Could you check a few things on this model? Use its own coordinates, in mm. A direction names the side the tool comes from. Round coordinates to 2 decimals unless told otherwise and drop trailing zeros. Order: outer loops, then holes, each group sorted by start corner. A loop starts at its lowest first (then second) coordinate and runs counter-clockwise, first axis right, second up. Notation, with made-up numbers: (5.25, 81) - (17.25, 81) arc R33 cw to (17.25, 113) - close; hole circle Ø3 at (59.5, 16). An arc over 180 degrees is marked (long way). Use one line per item in the form item = value.
from build123d import *

# Parameters (mm, degrees)
F0_R      = 5
F1_DEPTH  = 60
F3_W      = 309.3655258417
F3_H      = 284.4564542174
F4_DEPTH  = 37.5
F5_SIZE   = 12
F7_DEPTH  = 75
F9_R      = 20
F11_DEPTH = 86.9450472691
F8_R      = 5
F7_FACE_R = 5
F12_DEPTH = 22.5


# Not quite as in the source:
# - a feature names something its author has since deleted; it is built from what else it names


with BuildPart() as f1:
    # F0 (on Right) → F1 (new body, symmetric)
    with BuildSketch(Plane.YZ):
        Polygon((75, 130), (-75, 130), (-90, 130), (-108.526711476, 17.9430459013), (-58.9007476441, -170), (58.9007476441, -170), (108.526711476, 17.9430459013), (90, 130), align=None)
        with Locations((0, -117.917008698)):
            Circle(F0_R, mode=Mode.SUBTRACT)
        Circle(F0_R, mode=Mode.SUBTRACT)
    extrude(amount=F1_DEPTH, both=True)

    # F3 (on face) → F4 (cut, symmetric)
    with BuildSketch(Plane.YZ):
        with Locations((9.2283859849, -86.6799689829)):
            Rectangle(F3_W, F3_H)
    extrude(amount=F4_DEPTH, both=True, mode=Mode.SUBTRACT)

    # F5
    f5_edges = [f1.edges().sort_by_distance(p)[0] for p in [
        (-60, -99.263356, 73.971523),
        (-60, 99.263356, 73.971523),
        (60, -99.263356, 73.971523),
        (60, 99.263356, 73.971523),
    ]]
    chamfer(f5_edges, length=F5_SIZE)

    # F6 (on face) → F7 (join, through all)
    with BuildSketch(Plane.YZ.offset(-37.5)):
        Polygon((92.4365120253, -42.9936263649), (-92.4365120253, -42.9936263649), (-80.5341079321, -88.0703141729), (80.5341079321, -88.0703141729), align=None)
    extrude(amount=F7_DEPTH)

    # F9
    f9_edges = [f1.edges().sort_by_distance(p)[0] for p in [
        (-37.5, 0, 55.548258),
        (37.5, 0, 55.548258),
        (-37.5, 0, -42.993626),
        (37.5, 0, -42.993626),
    ]]
    fillet(f9_edges, radius=F9_R)

    # F10 (on face) → F11 (cut, through all)
    with BuildSketch(Plane.XY.offset(130)):
        Polygon((36.0373817384, 65.5976682901), (0, 65.5976682901), (-36.0373817384, 65.5976682901), (-36.0373817384, 0), (-36.0373817384, -65.5976682901), (0, -65.5976682901), (36.0373817384, -65.5976682901), (36.0373817384, 0), align=None)
    extrude(amount=-F11_DEPTH, mode=Mode.SUBTRACT)

    # F8 (on face) + F7_face (on face) → F12 (cut, through all)
    with BuildSketch(Plane.YZ.offset(60)):
        Polygon((25.2734031528, -88.0703141729), (-80.5341079321, -88.0703141729), (-58.9007476441, -170), (25.2734031528, -170), align=None)
        with Locations((0, -117.917008698)):
            Circle(F8_R, mode=Mode.SUBTRACT)
    with BuildSketch(Plane(origin=(37.5, 0, -126.978888881), x_dir=(0, -1, 0), z_dir=(-1, 0, 0))):
        Polygon((-80.5341079321, 38.9085747081), (-58.9007476441, -43.021111119), (58.9007476441, -43.021111119), (80.5341079321, 38.9085747081), align=None)
        with Locations((0, 9.061880183)):
            Circle(F7_FACE_R, mode=Mode.SUBTRACT)
    extrude(amount=-F12_DEPTH, dir=(1, 0, 0), mode=Mode.SUBTRACT)


solid = f1.part
Item 1: Imagine slicing it at B-B on y = 0. Please give me the cut outline in (x, z), plus the area to 3 significant figures.
Found:
outline = (-60, -170) - (-37.5, -170) - (-37.5, -122.92) - (-60, -122.92) - close; (-60, -112.92) - (-37.5, -112.92) - (-37.5, -88.07) - (60, -88.07) - (60, -5) - (37.5, -5) - (37.5, -22.99) arc R20 cw to (17.5, -42.99) - (-17.5, -42.99) arc R20 cw to (-37.5, -22.99) - (-37.5, -5) - (-60, -5) - close; (-60, 5) - (-37.5, 5) - (-37.5, 35.55) arc R20 cw to (-36.04, 43.06) - (-36.04, 130) - (-60, 130) - close; (36.04, 43.06) arc R20 cw to (37.5, 35.55) - (37.5, 5) - (60, 5) - (60, 130) - (36.04, 130) - close
area = 14,800 mm2
Item 2: I need wall thicknesses on L1, parallel to Z at x = -53.75, y = 0; L2, parallel to X at y = -5.5, z = 2; L3, parallel to X at y = -33, z = 48.5. Which ranges of each line are inside material? Lowest first, please.
Found:
L1 = -170 to -122.92, -112.92 to -5, 5 to 130
L2 = -60 to -37.5, 37.5 to 60
L3 = -60 to -36.04, 36.04 to 60
Item 3: Imagine slicing it at C-C on z = 0. Please give me the cut outline in (x, y), plus the area to 3 significant figures.
Found:
outline = (-60, -99.33) - (-55.6, -103.79) - (-37.5, -103.79) - (-37.5, -5) - (-60, -5) - close; (-60, 5) - (-37.5, 5) - (-37.5, 103.79) - (-55.6, 103.79) - (-60, 99.33) - close; (37.5, -103.79) - (55.6, -103.79) - (60, -99.33) - (60, -5) - (37.5, -5) - close; (37.5, 5) - (60, 5) - (60, 99.33) - (55.6, 103.79) - (37.5, 103.79) - close
area = 8,850 mm2
Item 4: If we mould it in two halves opening along X, with no side actions, what happens to faces 6 (the face through (-37.5, -2, 7)), 7 (the face through (49, 42, -170)), 8 (the face through (54.08, -95.12, 61.76)), 9 (the face through (-54.08, -95.12, 61.76))? For each: released by +X, released by -X, zero draft, split by the parting line, or undercut.
Found:
face_6 = undercut
face_7 = zero draft
face_8 = released by +X
face_9 = released by -X
Item 5: For faces 1 (the face through (37.5, 46, -128)), 2 (the face through (49, 25.273, -130)), 3 (the face through (-48.91, -1.08, -4.88)), 4 (the face through (-36.874, 1.479, 40.512)), 5 (the face through (-36.037, 1, 87)), which set-ups out of +Z, -Z, +X, -X, +Y, -Y let a thin tool reach every point of the face, with its end or its side?
Found:
face_1 = -Z, +Y, -Y
face_2 = -Z, +X, -Y
face_3 = +X, -X
face_4 = +Y, -Y
face_5 = +Z
Item 6: Will these pins go through, and if not, where does the flat tip stop? P1, Ø3, axis at x = 30.5, y = 33.5, coming from the +Z side; P2, Ø10.5, axis at x = 0, y = -35, coming from the +Z side; P3, Ø17.5, axis at x = 1, y = -83.5, coming from the -Z side; P4, Ø9, axis at y = 0, z = 0, coming from the -X side.
Found:
P1 = -36.77
P2 = -42.99
P3 = -88.07
P4 = through
Item 7: Imagine slicing it at D-D on y = 35. Please give me the cut outline in (x, z).
Found:
outline = (-60, -170) - (-37.5, -170) - (-37.5, -88.07) - (37.5, -88.07) - (37.5, -170) - (60, -170) - (60, 130) - (36.04, 130) - (36.04, 43.06) arc R20 cw to (37.5, 35.55) - (37.5, -22.99) arc R20 cw to (17.5, -42.99) - (-17.5, -42.99) arc R20 cw to (-37.5, -22.99) - (-37.5, 35.55) arc R20 cw to (-36.04, 43.06) - (-36.04, 130) - (-60, 130) - close
Item 8: Imagine slicing it at A-A on x = -12.5. Please give me the cut outline in (y, z), plus the area to 3 significant figures.
Found:
outline = (-102.31, 55.55) - (-65.6, 55.55) - (-65.6, 130) - (-90, 130) - close; (-92.44, -42.99) - (-80.53, -88.07) - (80.53, -88.07) - (92.44, -42.99) - close; (65.6, 55.55) - (102.31, 55.55) - (90, 130) - (65.6, 130) - close
area = 12,300 mm2
